Can you work these out from the model? Positions are in its coordinate system, mm. Face numbers are marked on the shaded views. A direction names the side the tool comes from. Give positions to 0.01 mm unless a question says otherwise; leave off trailing zeros. Loops run counter-clockwise (first coordinate to the right, second up) from the corner with the lowest first, then second, coordinate; pieces in that order, holes last. Notation, with made-up numbers: (28.25, 36.5) - (50.25, 36.5) arc R13 ccw to (50.25, 61.5) - close; hole circle Ø6 at (-3, 5.5). An arc over 180 degrees is marked (long way). Answer as a JSON object with one key per item and string values.
```python
from build123d import *

# Parameters (mm, degrees)
SKETCH_1_R               = 9
EXTRUDE_1_DEPTH          = 3.2
CUT_EXTRUDE_2_REACH      = 15.124
PATTERN_CIRCULAR_1_COUNT = 8
CUT_EXTRUDE_1_REACH      = 14.951
SKETCH_3_R               = 2
PATTERN_CIRCULAR_2_COUNT = 4
CUT_EXTRUDE_3_REACH      = 14.951
SKETCH_6_R               = 1.6


with BuildPart() as part:
    # 草图1 → 凸台-拉伸1 (new body)
    with BuildSketch(Plane(origin=(0, 0, 0), x_dir=(1, 0, 0), z_dir=(0, 1, 0))):
        with Locations(Location((0, 0, 0), (0, 0, 270))):
            Circle(SKETCH_1_R)
        with BuildLine():
            Line((-1.058300524, 1.2), (1.058300524, 1.2))
            ThreePointArc((1.058300524, 1.2), (0, -1.6), (-1.058300524, 1.2))
        make_face(mode=Mode.SUBTRACT)
    extrude(amount=EXTRUDE_1_DEPTH)

    # 草图4 → 切除-拉伸2 (cut, up to next)
    with BuildSketch(Plane(origin=(0, 3.2, 0), x_dir=(1, 0, 0), z_dir=(0, 1, 0)), mode=Mode.PRIVATE) as cut_extrude_2_sk1:
        with BuildLine():
            Line((-1.5, 8.874119675), (-0.599498979, 8.19962448))
            ThreePointArc((-0.599498979, 8.19962448), (0, 8), (0.599498979, 8.19962448))
            Line((0.599498979, 8.19962448), (1.5, 8.874119675))
            ThreePointArc((1.5, 8.874119675), (0, 9), (-1.5, 8.874119675))
        make_face()
    cut_extrude_2_tool1 = extrude(cut_extrude_2_sk1.sketch, amount=-CUT_EXTRUDE_2_REACH, mode=Mode.PRIVATE) & part.part
    cut_extrude_2 = cut_extrude_2_tool1.solids().sort_by_distance((0, 3.2, -8.590322))[0]
    add(cut_extrude_2, mode=Mode.SUBTRACT)

    # 阵列(圆周)1: 切除-拉伸2 ×8 about axis
    pattern_circular_1_axis = Axis((0, 0, 0), (0, 1, 0))
    for i in range(1, PATTERN_CIRCULAR_1_COUNT):
        add(cut_extrude_2.rotate(pattern_circular_1_axis, i * 360 / PATTERN_CIRCULAR_1_COUNT), mode=Mode.SUBTRACT)

    # 草图3 → 切除-拉伸1 (cut, up to next)
    with BuildSketch(Plane(origin=(0, 3.2, 0), x_dir=(1, 0, 0), z_dir=(0, 1, 0)), mode=Mode.PRIVATE) as cut_extrude_1_sk1:
        with Locations(Location((0, 5, 0), (0, 0, 270))):
            Circle(SKETCH_3_R)
    cut_extrude_1_tool1 = extrude(cut_extrude_1_sk1.sketch, amount=-CUT_EXTRUDE_1_REACH, mode=Mode.PRIVATE) & part.part
    cut_extrude_1 = cut_extrude_1_tool1.solids().sort_by_distance((0, 3.2, -5))[0]
    add(cut_extrude_1, mode=Mode.SUBTRACT)

    # 阵列(圆周)2: 切除-拉伸1 ×4 about axis
    pattern_circular_2_axis = Axis((0, 0, 0), (0, 1, 0))
    for i in range(1, PATTERN_CIRCULAR_2_COUNT):
        add(cut_extrude_1.rotate(pattern_circular_2_axis, i * 360 / PATTERN_CIRCULAR_2_COUNT), mode=Mode.SUBTRACT)

    # 草图5 → 切除-旋转1 (revolve, cut)
    with BuildSketch(Plane(origin=(0, 0, 0), x_dir=(0, 0, -1), z_dir=(1, 0, 0)), mode=Mode.PRIVATE) as cut_revolve_1_sk:
        Polygon((9.374119675, 2.82841307), (6.778765119, 3.2), (9.374119675, 3.2), align=None)
    cut_revolve_1 = revolve(cut_revolve_1_sk.sketch.rotate(Axis((0, 3.2, 0), (0, -1, 0)), 4.181624795), axis=Axis((0, 3.2, 0), (0, -1, 0)), mode=Mode.SUBTRACT)

    # 镜向1: 切除-旋转1 across plane
    add(cut_revolve_1.mirror(Plane.ZX.offset(1.6)), mode=Mode.SUBTRACT)

    # 草图6 → 切除-拉伸3 (cut, up to next)
    with BuildSketch(Plane(origin=(0, 3.2, 0), x_dir=(1, 0, 0), z_dir=(0, 1, 0)), mode=Mode.PRIVATE) as cut_extrude_3_sk1:
        with Locations(Location((0, 0, 0), (0, 0, 270))):
            Circle(SKETCH_6_R)
    cut_extrude_3_tool1 = extrude(cut_extrude_3_sk1.sketch, amount=-CUT_EXTRUDE_3_REACH, mode=Mode.PRIVATE) & part.part
    add(cut_extrude_3_tool1.solids().sort_by_distance((0, 3.2, 0))[0], mode=Mode.SUBTRACT)


solid = part.part
```
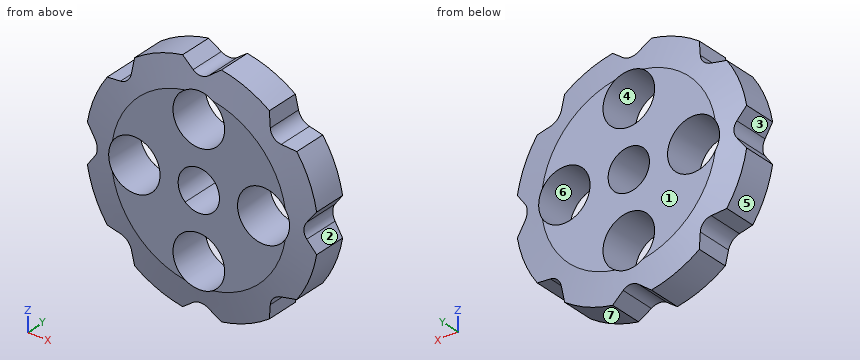
1) Which directions (+Z, -Z, +X, -X, +Y, -Y) give clear straight access to the entire face, cutting with the end or side of a thin tool? Please do the marked faces 1, 2 and 3.
Check sheet entries:
{"face 1": "+Z, -Z, +X, -X, +Y", "face 2": "+X, +Y, -Y", "face 3": "-X, +Y, -Y"}
2) Imagine slicing it at B-B on z = 0. Write out the boundary of the cut face in (x, y), and give its area (3 significant figures).
Check sheet entries:
{"outline": "(-8, 0.17) - (-7, 0.03) - (-7, 3.17) - (-8, 3.03) - close; (-3, 0) - (-1.6, 0) - (-1.6, 3.2) - (-3, 3.2) - close; (1.6, 0) - (3, 0) - (3, 3.2) - (1.6, 3.2) - close; (7, 0.03) - (8, 0.17) - (8, 3.03) - (7, 3.17) - close", "area": "14.9 mm2"}
3) I need wall thicknesses on L1, parallel to Z at x = -5, y = 1.95; L2, parallel to Z at x = 0.25, y = 2.35; L3, parallel to X at y = 2.2, z = -4.25. Which ranges of each line are inside material? Lowest first, please.
Check sheet entries:
{"L1": "-7.48 to -2, 2 to 7.48", "L2": "-8.03 to -6.98, -3.02 to -1.58, 1.58 to 3.02, 6.98 to 8.03", "L3": "-7.93 to -1.85, 1.85 to 7.93"}
4) Imagine slicing it at C-C on y = 1.45. Give the number of separate pieces and of enclosed holes in the cut face, and give its area (3 significant figures).
Check sheet entries:
{"separate pieces": "1", "enclosed holes": "5", "area": "182 mm2"}
5) I'm going to push flat-ended pins straight in: P1, Ø4.5, axis at x = 5, z = 0, coming from the +Y side; P2, Ø1, axis at x = 0, z = -0.5, coming from the +Y side; P3, Ø1, axis at y = 0.5, z = 0.5, coming from the -X side; P4, Ø1.5, axis at y = 1, z = -0.5, coming from the -X side. Where does each tip first touch, or does it pass through?
Check sheet entries:
{"P1": "y = 3.2", "P2": "through", "P3": "x = -8.5", "P4": "x = -8.69"}
6) Imagine slicing it at A-A on x = 0. Write out the boundary of the cut face in (y, z).
Check sheet entries:
{"outline": "(0, -3) - (3.2, -3) - (3.2, -1.6) - (0, -1.6) - close; (0, 1.6) - (3.2, 1.6) - (3.2, 3) - (0, 3) - close; (0.03, -7) - (0.17, -8) - (3.03, -8) - (3.17, -7) - close; (0.03, 7) - (3.17, 7) - (3.03, 8) - (0.17, 8) - close"}
7) If we mould it in two halves opening along X, with no side actions, what happens to the marked faces 4, 5, 6 and 7? For each: released by +X, released by -X, zero draft, split by the parting line, or undercut.
Check sheet entries:
{"face 4": "undercut", "face 5": "released by -X", "face 6": "undercut", "face 7": "released by +X"}
